Could you check a few things on this model? Use its own coordinates, in mm. A direction names the side the tool comes from. Round coordinates to 2 decimals unless told otherwise and drop trailing zeros. Loops run counter-clockwise (first coordinate to the right, second up) from the corner with the lowest first, then second, coordinate; pieces in that order, holes last.
from build123d import *

# Parameters (mm, degrees)
F0_W     = 127
F0_H     = 63.5
F1_DEPTH = 12.7
F2_DEPTH = 12.7
F3_R     = 5.08
F4_T     = -2.54


with BuildPart() as f1:
    # F0 (on Front) → F1 (new body)
    with BuildSketch(Plane.XZ):
        Rectangle(F0_W, F0_H)
    extrude(amount=F1_DEPTH)

    # F0 (on Front) → F2 (join)
    with BuildSketch(Plane.XZ):
        Rectangle(F0_W, F0_H)
    extrude(amount=F2_DEPTH)

    # F3
    f3_edges = [f1.edges().sort_by_distance(p)[0] for p in [
        (-63.5, -12.7, 0),
        (0, -12.7, -31.75),
        (63.5, -12.7, 0),
        (0, -12.7, 31.75),
        (63.5, -6.35, 31.75),
        (63.5, -6.35, -31.75),
        (-63.5, -6.35, -31.75),
        (-63.5, -6.35, 31.75),
    ]]
    fillet(f3_edges, radius=F3_R)

    # F4
    f4_openings = [f1.faces().sort_by_distance(p)[0] for p in [
        (0, 0, 0),
    ]]
    offset(amount=F4_T, openings=f4_openings)


solid = f1.part
Item 1: If I drill on line 1 along X through (y, z) = (-3.25, -21); line 2 along Z through (x, y) = (14, -3.5), over which ranges is the centre line in solid material (lowest first)?
Results list:
line 1: x = -63.5 to -60.96, 60.96 to 63.5
line 2: z = -31.75 to -29.21, 29.21 to 31.75
Item 2: For faces 5 (the flat face through (-1, -4, 29.21)), 6 (the flat face through (-1, -12.7, 0)), which set-ups out of +Z, -Z, +X, -X, +Y, -Y let a thin tool reach every point of the face, with its end or its side?
Results list:
face 5: +Y
face 6: +Z, -Z, +X, -X, -Y
Item 3: If we section it at A-A, the plane y = -4: Please give me the cut outline in (x, z), then the cut area to 3 significant figures.
Results list:
outline: (-63.5, -26.67) arc R5.08 ccw to (-58.42, -31.75) - (58.42, -31.75) arc R5.08 ccw to (63.5, -26.67) - (63.5, 26.67) arc R5.08 ccw to (58.42, 31.75) - (-58.42, 31.75) arc R5.08 ccw to (-63.5, 26.67) - close; hole (-60.96, -26.67) arc R2.54 ccw to (-58.42, -29.21) - (58.42, -29.21) arc R2.54 ccw to (60.96, -26.67) - (60.96, 26.67) arc R2.54 ccw to (58.42, 29.21) - (-58.42, 29.21) arc R2.54 ccw to (-60.96, 26.67) - close
area: 925 mm2
Item 4: We'd pull the mould along Z, two halves only. Please class faces 1 (the flat face through (-1, -4, 31.75)), 2 (the flat face through (-1, -10.16, 0)), 3 (the cylindrical face through (61.972, -3.863, -30.301)), 4 (the flat face through (-19, 0, -30)): released by +Z, released by -Z, zero draft, split by the parting line, or undercut.
Results list:
face 1: released by +Z
face 2: undercut
face 3: released by -Z
face 4: zero draft
Item 5: If we section it at C-C, the plane x = 23.5: Please give me the cut outline in (y, z).
Results list:
outline: (-12.7, -26.67) arc R5.08 ccw to (-7.62, -31.75) - (0, -31.75) - (0, -29.21) - (-7.62, -29.21) arc R2.54 cw to (-10.16, -26.67) - (-10.16, 26.67) arc R2.54 cw to (-7.62, 29.21) - (0, 29.21) - (0, 31.75) - (-7.62, 31.75) arc R5.08 ccw to (-12.7, 26.67) - close
Item 6: Will this pin go through, and if not, where does the flat tip stop? pin 1 (3 mm diameter, centred on x = -18.5, y = -10, fed in from +Z).
Results list:
pin 1: stops at z = 31.67
Item 7: If we section it at B-B, the plane z = 20: Please give me the cut outline in (x, y), then the cut area to 3 significant figures.
Results list:
outline: (-63.5, -7.62) arc R5.08 ccw to (-58.42, -12.7) - (58.42, -12.7) arc R5.08 ccw to (63.5, -7.62) - (63.5, 0) - (60.96, 0) - (60.96, -7.62) arc R2.54 cw to (58.42, -10.16) - (-58.42, -10.16) arc R2.54 cw to (-60.96, -7.62) - (-60.96, 0) - (-63.5, 0) - close
area: 366 mm2
